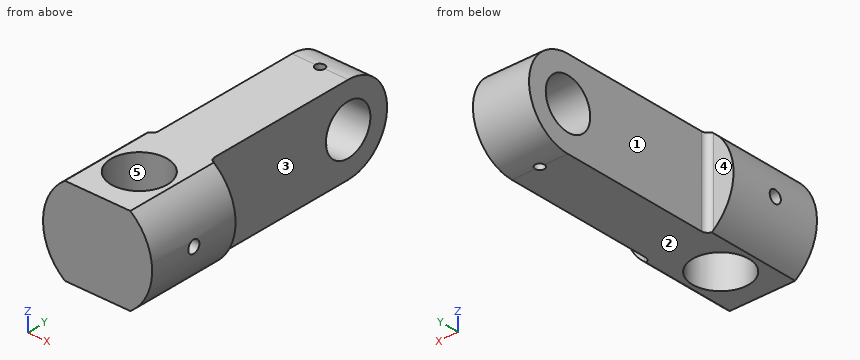
from build123d import *

# Parameters (mm, degrees)
SKETCH1_R               = 17.5
BOSS_EXTRUDE1_DEPTH     = 30
SKETCH2_W               = 18
SKETCH2_H               = 30.01666204
BOSS_EXTRUDE2_DEPTH     = 70
CUT_EXTRUDE1_DEPTH      = 104.01698889
CUT_EXTRUDE1_DEPTH_BACK = 104.01698889
CUT_EXTRUDE2_DEPTH      = 105.394683773
CUT_EXTRUDE2_DEPTH_BACK = 105.394683773
SKETCH4_R               = 8
CUT_EXTRUDE3_DEPTH      = 100.630567599
CUT_EXTRUDE3_DEPTH_BACK = 100.630567599
SKETCH6_R               = 9
FILLET1_R               = 2
CUT_EXTRUDE4_DEPTH      = 97.634621158
CUT_EXTRUDE4_DEPTH_BACK = 97.634621158
SKETCH7_R               = 2
CUT_EXTRUDE5_DEPTH      = 97.634621159
CUT_EXTRUDE5_DEPTH_BACK = 97.634621159
SKETCH8_R               = 1.5


with BuildPart() as part:
    # Sketch1 → Boss-Extrude1 (new body)
    with BuildSketch(Plane(origin=(0, 0, 0), x_dir=(1, 0, 0), z_dir=(0, 1, 0))):
        with Locations(Location((0, 0, 0), (0, 0, 270))):
            Circle(SKETCH1_R)
    extrude(amount=BOSS_EXTRUDE1_DEPTH)

    # Sketch2 → Boss-Extrude2 (add)
    with BuildSketch(Plane(origin=(0, 30, 0), x_dir=(1, 0, 0), z_dir=(0, 1, 0))):
        Rectangle(SKETCH2_W, SKETCH2_H)
    extrude(amount=BOSS_EXTRUDE2_DEPTH)

    # Sketch3 → Cut-Extrude1 (cut, two sides: drawn at the far end of the back side and taken through both)
    with BuildSketch(Plane.XZ.offset(-CUT_EXTRUDE1_DEPTH_BACK)):
        with BuildLine():
            Line((-10.5, -14), (10.5, -14))
            ThreePointArc((10.5, -14), (0, -17.5), (-10.5, -14))
        make_face()
        with BuildLine():
            Line((-10.5, 14), (10.5, 14))
            ThreePointArc((10.5, 14), (0, 17.5), (-10.5, 14))
        make_face()
    extrude(amount=CUT_EXTRUDE1_DEPTH + CUT_EXTRUDE1_DEPTH_BACK, mode=Mode.SUBTRACT)

    # Sketch4 → Cut-Extrude2 (cut, two sides: drawn at the far end of the back side and taken through both)
    with BuildSketch(Plane.ZY.offset(9).offset(-CUT_EXTRUDE2_DEPTH_BACK)):
        with Locations((0, 80)):
            Circle(SKETCH4_R)
        with BuildLine():
            Line((-14, 80), (-32.866525809, 80))
            Line((-32.866525809, 80), (-32.866525809, 110.116185887))
            Line((-32.866525809, 110.116185887), (25.904661095, 110.116185887))
            Line((25.904661095, 110.116185887), (25.904661095, 80))
            Line((25.904661095, 80), (14, 80))
            ThreePointArc((14, 80), (0, 94), (-14, 80))
        make_face()
    extrude(amount=CUT_EXTRUDE2_DEPTH + CUT_EXTRUDE2_DEPTH_BACK, mode=Mode.SUBTRACT)

    # Sketch6 → Cut-Extrude3 (cut, two sides: drawn at the far end of the back side and taken through both)
    with BuildSketch(Plane.XY.offset(-14).offset(-CUT_EXTRUDE3_DEPTH_BACK)):
        with Locations((0, 15)):
            Circle(SKETCH6_R)
    extrude(amount=CUT_EXTRUDE3_DEPTH + CUT_EXTRUDE3_DEPTH_BACK, mode=Mode.SUBTRACT)

    # Fillet1
    fillet1_edges = [part.edges().sort_by_distance(p)[0] for p in [
        (9, 30, 0),
        (-9, 30, 0),
    ]]
    fillet(fillet1_edges, radius=FILLET1_R)

    # Sketch7 → Cut-Extrude4 (cut, two sides: drawn at the far end of the back side and taken through both)
    with BuildSketch(Plane(origin=(0, 0, 0), x_dir=(0, 0, -1), z_dir=(1, 0, 0)).offset(-CUT_EXTRUDE4_DEPTH_BACK)):
        with Locations((0, 15)):
            Circle(SKETCH7_R)
    extrude(amount=CUT_EXTRUDE4_DEPTH + CUT_EXTRUDE4_DEPTH_BACK, mode=Mode.SUBTRACT)

    # Sketch8 → Cut-Extrude5 (cut, two sides: drawn at the far end of the back side and taken through both)
    with BuildSketch(Plane.XY.offset(-CUT_EXTRUDE5_DEPTH_BACK)):
        with Locations((0, 80)):
            Circle(SKETCH8_R)
    extrude(amount=CUT_EXTRUDE5_DEPTH + CUT_EXTRUDE5_DEPTH_BACK, mode=Mode.SUBTRACT)


solid = part.part
Input: part model. Units: mm. Frame: model coordinates. Face numbers are marked on the shaded views. A direction names the side the tool comes from. Coordinates: 2 decimals unless noted, no trailing zeros. Loops run counter-clockwise (first coordinate to the right, second up) from the corner with the lowest first, then second, coordinate; pieces in that order, holes last.
(1) Section A-A on z = 0. Return the cut outline in (x, y), then the cut area to 3 significant figures.
(2) Material intervals for probe 1 along X at (y, z) = (80, -11.75); probe 2 along Z at (x, y) = (14, 15); probe 3 along Y at (x, z) = (0, -9.5), sorted ascending.
(3) Section D-D on x = 0. Return the cut outline in (y, z).
(4) First-contact query: pin 1 Ø5 at (y, z) = (42.5, 6) entering from -X; pin 2 Ø6 at (y, z) = (51, -10.5) entering from +X; pin 3 Ø1.5 at (x, z) = (-7.5, -4.5) entering from -Y; pin 4 Ø3.5 at (x, z) = (14.5, -2) entering from +Y. Flat tips, straight axial feed; report the tip coordinate or a pass-through.
(5) Section B-B on z = 4. Return the cut outline in (x, y), then the cut area to 3 significant figures.
(6) Pull-direction query (Y, two-part tool) for the marked faces 3, 4 and 5; classes: released by +Y, released by -Y, zero draft, split by the parting line, or undercut.
(7) Set-up query: the marked faces 1 and 2. Return all of +Z, -Z, +X, -X, +Y, -Y with unobstructed straight access to the full face (end or side cutting, diameter ignored); none if empty.
(8) Section C-C on x = 4.5. Return the cut outline in (y, z), then the cut area to 3 significant figures.
Data:
1. outline: (-17.5, 0) - (17.5, 0) - (17.5, 13) - (8.77, 13) arc R9 cw to (-8.77, 13) - (-17.5, 13) - close; (-17.5, 17) - (-8.77, 17) arc R9 cw to (8.77, 17) - (17.5, 17) - (17.5, 30) - (11, 30) arc R2 cw to (9, 32) - (9, 72) - (-9, 72) - (-9, 32) arc R2 cw to (-11, 30) - (-17.5, 30) - close; (-9, 88) - (9, 88) - (9, 94) - (-9, 94) - close
1. area: 1,590 mm2
2. probe 1: x = -9 to -1.5, 1.5 to 9
2. probe 2: z = -10.5 to -2, 2 to 10.5
2. probe 3: y = 0 to 6, 24 to 78.5, 81.5 to 90.28
3. outline: (0, -14) - (6, -14) - (6, 14) - (0, 14) - close; (24, -14) - (78.5, -14) - (78.5, -7.86) arc R8 cw to (78.5, 7.86) - (78.5, 14) - (24, 14) - close; (81.5, -13.92) arc R14 ccw to (81.5, 13.92) - (81.5, 7.86) arc R8 cw to (81.5, -7.86) - close
4. pin 1: stops at x = -9
4. pin 2: stops at x = 9
4. pin 3: stops at y = 0
4. pin 4: stops at y = 30
5. outline: (-17.04, 0) - (17.04, 0) - (17.04, 30) - (11, 30) arc R2 cw to (9, 32) - (9, 73.07) - (-9, 73.07) - (-9, 32) arc R2 cw to (-11, 30) - (-17.04, 30) - close; (-9, 86.93) - (9, 86.93) - (9, 93.42) - (-9, 93.42) - close; hole circle Ø18 at (0, 15)
5. area: 1,660 mm2
6. face 3: zero draft
6. face 4: released by +Y
6. face 5: undercut
7. face 1: +Z, -Z, -X, +Y
7. face 2: -Z, +X, -X, +Y, -Y
8. outline: (0, -14) - (7.21, -14) - (7.21, 14) - (0, 14) - close; (22.79, -14) - (80, -14) arc R14 ccw to (80, 14) - (22.79, 14) - close; hole circle Ø16 at (80, 0)
8. area: 1,910 mm2
